from build123d import *

# Parameters (mm, degrees)
ESQUISSE1_W             = 230
ESQUISSE1_H             = 270
BOSS_EXTRU_1_DEPTH      = 5
ESQUISSE2_R             = 2
ESQUISSE2_R_2           = 1.75
ESQUISSE2_R_3           = 1.5
ENL_V_MAT_EXTRU_1_DEPTH = 5
COQUE3_T                = -1.5
ESQUISSE3_R             = 4.5
ESQUISSE3_R_2           = 2.5
BOSS_EXTRU_3_DEPTH      = 25
ESQUISSE4_W             = 1
ESQUISSE4_H             = 267
BOSS_EXTRU_4_DEPTH      = 3.5
ESQUISSE5_W             = 225
ESQUISSE5_H             = 1
ESQUISSE5_H_2           = 2.9
BOSS_EXTRU_10_DEPTH     = 3.5
ESQUISSE7_W             = 2
ESQUISSE7_H             = 100
BOSS_EXTRU_11_DEPTH     = 25
ESQUISSE8_W             = 230
ESQUISSE8_H             = 270
ESQUISSE8_W_2           = 225
ESQUISSE8_H_2           = 263.1
BOSS_EXTRU_12_DEPTH     = 25
ESQUISSE13_W            = 17
ESQUISSE13_H            = 55
ENL_V_MAT_EXTRU_4_DEPTH = 10
ESQUISSE16_W            = 7.5
ESQUISSE16_H            = 5.6
BOSS_EXTRU_13_DEPTH     = 28.5
ESQUISSE17_R            = 2
ENL_V_MAT_EXTRU_5_DEPTH = 213.83636063


with BuildPart() as part:
    # Esquisse1 → Boss.-Extru.1 (new body)
    with BuildSketch(Plane.XY):
        with Locations((0, -41.5625)):
            Rectangle(ESQUISSE1_W, ESQUISSE1_H)
    extrude(amount=BOSS_EXTRU_1_DEPTH)

    # Esquisse2 → Enlèv. mat.-Extru.1 (cut)
    with BuildSketch(Plane.XY.offset(5)):
        with Locations((-104, -163.5625)):
            Circle(ESQUISSE2_R)
        with Locations(Location((-104, 9.4375, 0), (0, 0, 180))):
            Circle(ESQUISSE2_R)
        with Locations((104.5, 82.9375)):
            Circle(ESQUISSE2_R_2)
        with Locations((24.5, 82.9375)):
            Circle(ESQUISSE2_R_2)
        with Locations(Location((24.5, 39.9375, 0), (0, 0, 180))):
            Circle(ESQUISSE2_R_2)
        with Locations(Location((104.5, 39.9375, 0), (0, 0, 180))):
            Circle(ESQUISSE2_R_2)
        with Locations((-87.5, 85.9375)):
            Circle(ESQUISSE2_R_3)
        with Locations(Location((-29.5, 85.9375, 0), (0, 0, 180))):
            Circle(ESQUISSE2_R_3)
        with Locations((8.5, 67.4375)):
            Circle(ESQUISSE2_R_3)
        with Locations(Location((-12.5, 67.4375, 0), (0, 0, 180))):
            Circle(ESQUISSE2_R_3)
        with Locations((-12.5, 79.9375)):
            Circle(ESQUISSE2_R_3)
        with Locations(Location((8.5, 79.9375, 0), (0, 0, 180))):
            Circle(ESQUISSE2_R_3)
        with Locations(Location((101, -163.5625, 0), (0, 0, 180))):
            Circle(ESQUISSE2_R)
        with Locations((101, 9.4375)):
            Circle(ESQUISSE2_R)
        with Locations(Location((-87.5, 36.9375, 0), (0, 0, 180))):
            Circle(ESQUISSE2_R_3)
        with Locations((-29.5, 36.9375)):
            Circle(ESQUISSE2_R_3)
    extrude(amount=-ENL_V_MAT_EXTRU_1_DEPTH, mode=Mode.SUBTRACT)

    # Coque3
    coque3_openings = [part.faces().sort_by_distance(p)[0] for p in [
        (-0.011238138, -41.697281592, 5),
    ]]
    offset(amount=COQUE3_T, openings=coque3_openings, kind=Kind.INTERSECTION)

    # Esquisse3 → Boss.-Extru.3 (add)
    # profile 1 of 4: a face of its own
    with BuildSketch(Plane.XY.offset(1.5)):
        with Locations(Location((-104, 9.4375, 0), (0, 0, 180))):
            Circle(ESQUISSE3_R)
        with Locations(Location((-104, 9.4375, 0), (0, 0, 180))):
            Circle(ESQUISSE3_R_2, mode=Mode.SUBTRACT)
    # profile 2 of 4: a face of its own
    with BuildSketch(Plane.XY.offset(1.5)):
        with Locations(Location((-104, -163.5625, 0), (0, 0, 180))):
            Circle(ESQUISSE3_R)
        with Locations(Location((-104, -163.5625, 0), (0, 0, 180))):
            Circle(ESQUISSE3_R_2, mode=Mode.SUBTRACT)
    # profile 3 of 4: a face of its own
    with BuildSketch(Plane.XY.offset(1.5)):
        with Locations(Location((101, -163.5625, 0), (0, 0, 180))):
            Circle(ESQUISSE3_R)
        with Locations(Location((101, -163.5625, 0), (0, 0, 180))):
            Circle(ESQUISSE3_R_2, mode=Mode.SUBTRACT)
    # profile 4 of 4: a face of its own
    with BuildSketch(Plane.XY.offset(1.5)):
        with Locations(Location((101, 9.4375, 0), (0, 0, 180))):
            Circle(ESQUISSE3_R)
        with Locations(Location((101, 9.4375, 0), (0, 0, 180))):
            Circle(ESQUISSE3_R_2, mode=Mode.SUBTRACT)
    extrude(amount=BOSS_EXTRU_3_DEPTH)

    # Esquisse4 → Boss.-Extru.4 (add)
    with BuildSketch(Plane.XY.offset(1.5)):
        with Locations((-113, -41.5625)):
            Rectangle(ESQUISSE4_W, ESQUISSE4_H)
        with Locations((113, -41.5625)):
            Rectangle(ESQUISSE4_W, ESQUISSE4_H)
    extrude(amount=BOSS_EXTRU_4_DEPTH)

    # Esquisse5 → Boss.-Extru.10 (add)
    with BuildSketch(Plane.XY.offset(1.5)):
        with Locations((0, 91.4375)):
            Rectangle(ESQUISSE5_W, ESQUISSE5_H)
        with Locations((0, -173.6125)):
            Rectangle(ESQUISSE5_W, ESQUISSE5_H_2)
    extrude(amount=BOSS_EXTRU_10_DEPTH)

    # Esquisse7 → Boss.-Extru.11 (add)
    with BuildSketch(Plane.XY.offset(1.5)):
        with Locations((0, -72.1625)):
            Rectangle(ESQUISSE7_W, ESQUISSE7_H)
        with Locations((-55, -72.1625)):
            Rectangle(ESQUISSE7_W, ESQUISSE7_H)
        with Locations((55, -72.1625)):
            Rectangle(ESQUISSE7_W, ESQUISSE7_H)
    extrude(amount=BOSS_EXTRU_11_DEPTH)

    # Esquisse8 → Boss.-Extru.12 (add)
    with BuildSketch(Plane.XY.offset(5)):
        with Locations((0, -41.5625)):
            Rectangle(ESQUISSE8_W, ESQUISSE8_H)
        with Locations((0, -40.6125)):
            Rectangle(ESQUISSE8_W_2, ESQUISSE8_H_2, mode=Mode.SUBTRACT)
    extrude(amount=BOSS_EXTRU_12_DEPTH)

    # Esquisse13 → Enlèv. mat.-Extru.4 (cut)
    with BuildSketch(Plane(origin=(-112.5, 0, 0), x_dir=(0, 0, -1), z_dir=(1, 0, 0))):
        with Locations((-14.5, 61.4375)):
            Rectangle(ESQUISSE13_W, ESQUISSE13_H)
    extrude(amount=-ENL_V_MAT_EXTRU_4_DEPTH, mode=Mode.SUBTRACT)

    # Esquisse16 → Boss.-Extru.13 (add)
    with BuildSketch(Plane.XY.offset(1.5)):
        with Locations((-108.75, -169.3625)):
            Rectangle(ESQUISSE16_W, ESQUISSE16_H)
        with Locations((108.75, -169.3625)):
            Rectangle(ESQUISSE16_W, ESQUISSE16_H)
    extrude(amount=BOSS_EXTRU_13_DEPTH)

    # Esquisse17 → Enlèv. mat.-Extru.5 (cut, through all)
    with BuildSketch(Plane.XY.offset(30)):
        with Locations((-110, -171.5625)):
            Circle(ESQUISSE17_R)
        with Locations((110, -171.5625)):
            Circle(ESQUISSE17_R)
    extrude(amount=-ENL_V_MAT_EXTRU_5_DEPTH, mode=Mode.SUBTRACT)


solid = part.part
Design review of the part built by this model. Coordinates are the model's own, in mm. A direction names the side the tool comes from. Coordinates: 2 decimals unless noted, no trailing zeros. Loops run counter-clockwise (first coordinate to the right, second up) from the corner with the lowest first, then second, coordinate; pieces in that order, holes last. Notation, with made-up numbers: (25, 14.25) - (82, 14.25) arc R21 cw to (82, 31.25) - close; hole circle Ø6 at (-21, 29.5). An arc over 180 degrees is marked (long way). Use CSV: the item, a comma, the result in double quotes. Start each with the question number.
1. Clearance check with flat-ended pins moving along their axes: pin 1 (1.5 mm diameter, centred on x = 89.5, y = 57, fed in from +Z); pin 2 (10 mm diameter, centred on x = -55, y = -107.5, fed in from +Z); pin 3 (5 mm diameter, centred on x = -30.5, y = 87, fed in from +Z). State where each tip first meets the part, or that it passes through.
2. To check wall thickness, follow probe 1 along X at (y, z) = (-120.5, 20.5); probe 2 along Y at (x, z) = (104.5, 1.25); probe 3 along Y at (x, z) = (-104, 3.15). State the ranges of each line that lie inside material, in increasing order.
3. Add section A-A on y = 0. Give the boundary of the cut face in (x, z), plus the area to 4 significant figures.
4. Add section C-C on y = -86.5. Give the boundary of the cut face in (x, z), plus the area to 4 significant figures.
5. For faces 1 (the flat face through (-115, -43, 15)), 2 (the flat face through (10, 66, 5)), list the 3-axis set-ups (+Z, -Z, +X, -X, +Y, -Y) from which the entire face can be reached by the end or side of a thin tool; tool diameter is ignored.
6. Add section D-D on z = 14.5. Count the separate pieces of the cut face and the enclosed holes in it, plus the area to 3 significant figures.
7. Add section B-B on x = 42.5. Give the boundary of the cut face in (y, z), plus the area to 3 significant figures.
8. Mouldability with a two-part tool opening along X and no side actions: class faces 3 (the flat face through (-2, 93.438, 15)), 4 (the flat face through (-105.9, -161.6, 26.5)), 5 (the flat face through (115, -43, 15)) as released by +X, released by -X, zero draft, split by the parting line, or undercut.
Resolved:
1,pin 1,"z = 1.5"
1,pin 2,"z = 26.5"
1,pin 3,"z = 5"
2,probe 1,"-115 to -112.5, -56 to -54, -1 to 1, 54 to 56, 112.5 to 115"
2,probe 2,"-176.56 to 38.19, 41.69 to 81.19, 84.69 to 93.44"
2,probe 3,"-176.56 to -172.16, -168.06 to -165.56, -161.56 to -159.06, 4.94 to 7.44, 11.44 to 13.94, 90.94 to 93.44"
3,outline,"(-115, 0) - (115, 0) - (115, 30) - (112.5, 30) - (112.5, 1.5) - (-112.5, 1.5) - (-112.5, 30) - (-115, 30) - close"
3,area,"487.5 mm2"
4,outline,"(-115, 0) - (115, 0) - (115, 30) - (112.5, 30) - (112.5, 1.5) - (56, 1.5) - (56, 26.5) - (54, 26.5) - (54, 1.5) - (1, 1.5) - (1, 26.5) - (-1, 26.5) - (-1, 1.5) - (-54, 1.5) - (-54, 26.5) - (-56, 26.5) - (-56, 1.5) - (-112.5, 1.5) - (-112.5, 30) - (-115, 30) - close"
4,area,"637.5 mm2"
5,face 1,"+Z, -Z, -X, +Y, -Y"
5,face 2,"+Z"
6,separate pieces,"7"
6,enclosed holes,"6"
6,area,"3,600 mm2"
7,outline,"(-176.56, 0) - (93.44, 0) - (93.44, 30) - (90.94, 30) - (90.94, 1.5) - (-172.16, 1.5) - (-172.16, 30) - (-176.56, 30) - close"
7,area,"602 mm2"
8,face 3,"zero draft"
8,face 4,"undercut"
8,face 5,"released by +X"
